```python
from build123d import *

# Parameters (mm, degrees)
MODEL_R               = 4.250003312
MODEL_R_2             = 2.750739051
MODEL_R_3             = 2
TABAN_FLAN_1_DEPTH    = 4
IZIM1_W               = 33.261087109
IZIM1_H               = 28.852991227
SEKME1_DEPTH          = 4
IZIM4_R               = 14
KES_EKSTR_ZYON1_DEPTH = 10
IZIM5_R               = 6
KES_EKSTR_ZYON2_DEPTH = 10
RADYUS1_R             = 3
IZIM6_R               = 10.255106093
IZIM6_R_2             = 3.797139687
SEKME2_DEPTH          = 4
IZIM9_R               = 6
KES_EKSTR_ZYON3_DEPTH = 10
RADYUS2_R             = 4


# Sheet-metal steps are written as plain solids
with BuildPart() as part:
    # Model → Taban-Flanş1 (new body)
    with BuildSketch(Plane.XY):
        with BuildLine():
            add(Edge.make_bspline(
                [(3109.63786856, 2115.37754708), (3122.91316856, 2098.00144708), (3141.75296856, 2085.65664708), (3166.15706856, 2078.66474708)],
                knots=[0, 0, 0, 0, 0.026315789, 0.026315789, 0.026315789, 0.026315789], degree=3))
            add(Edge.make_bspline(
                [(3166.15706856, 2078.66474708), (3179.36946856, 2065.40354708), (3192.38586856, 2064.16554708), (3205.20626856, 2074.95084708)],
                knots=[0.052631579, 0.052631579, 0.052631579, 0.052631579, 0.078947368, 0.078947368, 0.078947368, 0.078947368], degree=3))
            add(Edge.make_bspline(
                [(3205.20626856, 2074.95084708), (3212.44426856, 2078.61404708), (3218.99666856, 2080.89554708), (3224.86356856, 2081.79514708)],
                knots=[0.105263158, 0.105263158, 0.105263158, 0.105263158, 0.131578947, 0.131578947, 0.131578947, 0.131578947], degree=3))
            add(Edge.make_bspline(
                [(3224.86356856, 2081.79514708), (3233.64336856, 2084.49734708), (3242.39766856, 2089.13084708), (3251.12626856, 2095.69584708)],
                knots=[0.157894737, 0.157894737, 0.157894737, 0.157894737, 0.184210526, 0.184210526, 0.184210526, 0.184210526], degree=3))
            add(Edge.make_bspline(
                [(3251.12626856, 2095.69584708), (3263.93226856, 2104.28284708), (3275.34806856, 2118.40454708), (3281.50066856, 2133.81654708)],
                knots=[0.210526316, 0.210526316, 0.210526316, 0.210526316, 0.236842105, 0.236842105, 0.236842105, 0.236842105], degree=3))
            add(Edge.make_bspline(
                [(3281.50066856, 2133.81654708), (3281.95096856, 2134.68714708), (3281.66796856, 2135.06734708), (3280.65166856, 2134.95694708)],
                knots=[0.263157895, 0.263157895, 0.263157895, 0.263157895, 0.289473684, 0.289473684, 0.289473684, 0.289473684], degree=3))
            add(Edge.make_bspline(
                [(3280.65166856, 2134.95694708), (3276.72366856, 2135.05064708), (3267.28426856, 2132.56494708), (3268.20996856, 2138.83004708)],
                knots=[0.315789474, 0.315789474, 0.315789474, 0.315789474, 0.342105263, 0.342105263, 0.342105263, 0.342105263], degree=3))
            add(Edge.make_bspline(
                [(3268.20996856, 2138.83004708), (3268.29816856, 2144.94904708), (3268.34226856, 2148.00864708)],
                knots=[0.368421053, 0.368421053, 0.368421053, 0.394736842, 0.394736842, 0.394736842], degree=2))
            add(Edge.make_bspline(
                [(3268.34226856, 2148.00864708), (3268.05746856, 2149.32424708), (3267.22186856, 2149.86364708), (3265.83536856, 2149.62684708)],
                knots=[0.421052632, 0.421052632, 0.421052632, 0.421052632, 0.447368421, 0.447368421, 0.447368421, 0.447368421], degree=3))
            add(Edge.make_bspline(
                [(3265.83536856, 2149.62684708), (3252.29706856, 2139.83354708), (3245.67386856, 2134.76664708), (3245.96566856, 2134.42624708)],
                knots=[0.473684211, 0.473684211, 0.473684211, 0.473684211, 0.5, 0.5, 0.5, 0.5], degree=3))
            add(Edge.make_bspline(
                [(3245.96566856, 2134.42624708), (3252.10236856, 2127.74094708), (3255.17056856, 2124.39824708)],
                knots=[0.526315789, 0.526315789, 0.526315789, 0.552631579, 0.552631579, 0.552631579], degree=2))
            add(Edge.make_bspline(
                [(3255.17056856, 2124.39824708), (3241.72096856, 2116.62674708), (3227.91756856, 2111.32994708), (3213.76056856, 2108.50784708)],
                knots=[0.578947368, 0.578947368, 0.578947368, 0.578947368, 0.605263158, 0.605263158, 0.605263158, 0.605263158], degree=3))
            add(Edge.make_bspline(
                [(3213.76056856, 2108.50784708), (3203.77946856, 2108.56904708), (3198.07446856, 2109.89254708), (3196.41116856, 2110.73614708)],
                knots=[0.631578947, 0.631578947, 0.631578947, 0.631578947, 0.657894737, 0.657894737, 0.657894737, 0.657894737], degree=3))
            add(Edge.make_bspline(
                [(3196.41116856, 2110.73614708), (3189.81546856, 2113.01174708), (3183.42196856, 2112.68434708), (3177.23076856, 2109.75424708)],
                knots=[0.684210526, 0.684210526, 0.684210526, 0.684210526, 0.710526316, 0.710526316, 0.710526316, 0.710526316], degree=3))
            add(Edge.make_bspline(
                [(3177.23076856, 2109.75424708), (3158.79236856, 2105.21744708), (3138.82946856, 2115.68974708), (3122.63636856, 2123.49564708)],
                knots=[0.736842105, 0.736842105, 0.736842105, 0.736842105, 0.763157895, 0.763157895, 0.763157895, 0.763157895], degree=3))
            add(Edge.make_bspline(
                [(3122.63636856, 2123.49564708), (3121.05686856, 2125.98834708), (3120.33186856, 2127.40314708), (3120.46116856, 2127.73984708)],
                knots=[0.789473684, 0.789473684, 0.789473684, 0.789473684, 0.815789474, 0.815789474, 0.815789474, 0.815789474], degree=3))
            add(Edge.make_bspline(
                [(3120.46116856, 2127.73984708), (3120.65286856, 2134.03014708), (3118.79596856, 2137.76174708), (3114.89056856, 2138.93464708)],
                knots=[0.842105263, 0.842105263, 0.842105263, 0.842105263, 0.868421053, 0.868421053, 0.868421053, 0.868421053], degree=3))
            add(Edge.make_bspline(
                [(3114.89056856, 2138.93464708), (3107.86456856, 2140.79974708), (3103.26626856, 2138.32384708), (3101.09596856, 2131.50664708)],
                knots=[0.894736842, 0.894736842, 0.894736842, 0.894736842, 0.921052632, 0.921052632, 0.921052632, 0.921052632], degree=3))
            add(Edge.make_bspline(
                [(3101.09596856, 2131.50664708), (3101.31076856, 2127.06704708), (3104.15806856, 2121.69074708), (3109.63786856, 2115.37754708)],
                knots=[0.947368421, 0.947368421, 0.947368421, 0.947368421, 1, 1, 1, 1], degree=3))
        make_face()
        with Locations((3110.978473341, 2130.220867466)):
            Circle(MODEL_R, mode=Mode.SUBTRACT)
        with Locations((3151.181278155, 2092.882262914)):
            Circle(MODEL_R_2, mode=Mode.SUBTRACT)
        with Locations((3131.238292653, 2113.390554749)):
            Circle(MODEL_R_3, mode=Mode.SUBTRACT)
        with Locations((3124.175950785, 2106.066377098)):
            Circle(MODEL_R_3, mode=Mode.SUBTRACT)
        with Locations((3266.454212243, 2126.936459372)):
            Circle(MODEL_R_3, mode=Mode.SUBTRACT)
        with Locations((3259.391870375, 2119.612281721)):
            Circle(MODEL_R_3, mode=Mode.SUBTRACT)
        with Locations((3228.404290977, 2099.075593739)):
            Circle(MODEL_R_3, mode=Mode.SUBTRACT)
        with Locations((3221.341949109, 2091.751416088)):
            Circle(MODEL_R_3, mode=Mode.SUBTRACT)
        with BuildLine():
            add(Edge.make_bspline(
                [(3202.10906856, 2089.91944708), (3202.10906856, 2097.65144708), (3195.84106856, 2103.91944708), (3188.10906856, 2103.91944708)],
                knots=[0, 0, 0, 0, 0.2, 0.2, 0.2, 0.2], degree=3))
            add(Edge.make_bspline(
                [(3188.10906856, 2103.91944708), (3180.37706856, 2103.91954708), (3174.10906856, 2097.65154708), (3174.10906856, 2089.91954708)],
                knots=[0.2, 0.2, 0.2, 0.2, 0.4, 0.4, 0.4, 0.4], degree=3))
            add(Edge.make_bspline(
                [(3174.10906856, 2089.91954708), (3174.10906856, 2082.18754708), (3180.37696856, 2075.91954708), (3188.10896856, 2075.91944708)],
                knots=[0.4, 0.4, 0.4, 0.4, 0.6, 0.6, 0.6, 0.6], degree=3))
            add(Edge.make_bspline(
                [(3188.10896856, 2075.91944708), (3195.84096856, 2075.91944708), (3202.10896856, 2082.18744708), (3202.10906856, 2089.91944708)],
                knots=[0.6, 0.6, 0.6, 0.6, 1, 1, 1, 1], degree=3))
        make_face(mode=Mode.SUBTRACT)
    extrude(amount=-TABAN_FLAN_1_DEPTH)

    # Çizim1 → Sekme1 (add)
    with BuildSketch(Plane.XY):
        with Locations((3187.445358668, 2090.033249542)):
            Rectangle(IZIM1_W, IZIM1_H)
    extrude(amount=-SEKME1_DEPTH)

    # Çizim4 → Kes-Ekstrüzyon1 (cut)
    with BuildSketch(Plane.XY):
        with Locations((3188.176183509, 2090.122283307)):
            Circle(IZIM4_R)
    extrude(amount=-KES_EKSTR_ZYON1_DEPTH, mode=Mode.SUBTRACT)

    # Çizim5 → Kes-Ekstrüzyon2 (cut)
    with BuildSketch(Plane(origin=(0, 0, -4), x_dir=(-1, 0, 0), z_dir=(0, 0, -1))):
        with Locations((-3238.176183509, 2102.122283307)):
            Circle(IZIM5_R)
    extrude(amount=-KES_EKSTR_ZYON2_DEPTH, mode=Mode.SUBTRACT)

    # Radyus1
    radyus1_edges = [part.edges().sort_by_distance(p)[0] for p in [
        (3255.17056856, 2124.39824708, -2),
    ]]
    fillet(radyus1_edges, radius=RADYUS1_R)

    # Çizim6 → Sekme2 (add)
    with BuildSketch(Plane(origin=(0, 0, -4), x_dir=(-1, 0, 0), z_dir=(0, 0, -1))):
        with Locations((-3110.978473341, 2130.220867466)):
            Circle(IZIM6_R)
        with Locations((-3110.978473341, 2130.220867466)):
            Circle(IZIM6_R_2, mode=Mode.SUBTRACT)
    extrude(amount=-SEKME2_DEPTH)

    # Çizim9 → Kes-Ekstrüzyon3 (cut)
    with BuildSketch(Plane(origin=(0, 0, -4), x_dir=(-1, 0, 0), z_dir=(0, 0, -1))):
        with Locations((-3110.978473341, 2130.220867466)):
            Circle(IZIM9_R)
    extrude(amount=-KES_EKSTR_ZYON3_DEPTH, mode=Mode.SUBTRACT)

    # Radyus2
    radyus2_edges = [part.edges().sort_by_distance(p)[0] for p in [
        (3122.63636856, 2123.49564708, -2),
        (3120.680098466, 2126.897364658, -2),
    ]]
    fillet(radyus2_edges, radius=RADYUS2_R)


solid = part.part
```
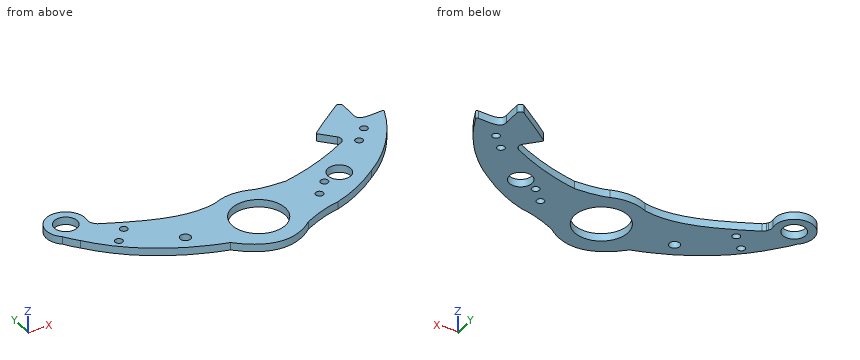
Geometry check sheet. Reference: the model listing, model coordinates, mm. Round coordinates to 2 decimals unless told otherwise and drop trailing zeros. Use a Markdown table: item, result. Add a question column.
1) Gauge pin test, flat ends, axial feed: P1, Ø4.5, axis at x = 3151.18, y = 2092.88, coming from the -Z side; P2, Ø15.5, axis at x = 3238.18, y = 2102.12, coming from the -Z side. Record the tip position at first contact, or that the pin passes through.
2) Thickness scan on line 1 along X through (y, z) = (2094, -1.8); line 2 along X through (y, z) = (2120, -0.85); line 3 along X through (y, z) = (2127, -1.25). Record the ranges inside material, lowest first.
3) Section check A-A (z = -2.1). Count the separate pieces of the cut face and the enclosed holes in it, then the cut area to 3 significant figures.
Established:
| question | item | result |
|---|---|---|
| 1 | P1 | through |
| 1 | P2 | z = -4 |
| 2 | line 1 | 3132.41 to 3148.67, 3153.69 to 3174.72, 3201.63 to 3248.81 |
| 2 | line 2 | 3105.98 to 3129.87, 3246.99 to 3257.43, 3261.35 to 3274.39 |
| 2 | line 3 | 3101.24 to 3105.92, 3116.04 to 3120.97, 3252.77 to 3264.46, 3268.45 to 3278.4 |
| 3 | separate pieces | 1 |
| 3 | enclosed holes | 10 |
| 3 | area | 4,540 mm2 |
